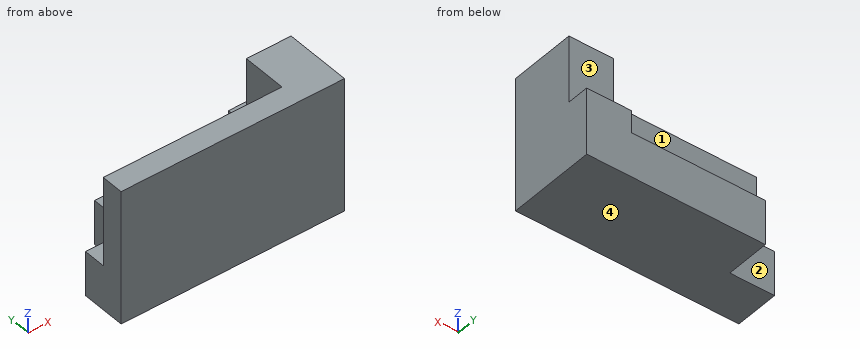
from build123d import *

# Parameters (mm, degrees)
SALIENTE_EXTRUIR1_DEPTH = 10
CROQUIS1_3_W            = 20
CROQUIS1_3_H            = 30
SALIENTE_EXTRUIR2_DEPTH = 30
SALIENTE_EXTRUIR3_DEPTH = 40
CROQUIS1_5_W            = 20
CROQUIS1_5_H            = 20
SALIENTE_EXTRUIR4_DEPTH = 20


with BuildPart() as part:
    # Croquis1 → Saliente-Extruir1 (new body)
    with BuildSketch(Plane(origin=(0, 0, 0), x_dir=(1, 0, 0), z_dir=(0, 1, 0))):
        Polygon((-30, 10), (-50, 10), (-50, -30), (30, -30), (30, 0), (30, 10), align=None)
    extrude(amount=SALIENTE_EXTRUIR1_DEPTH)

    # Croquis1<3> → Saliente-Extruir2 (add)
    with BuildSketch(Plane(origin=(0, 0, 0), x_dir=(1, 0, 0), z_dir=(0, 1, 0))):
        with Locations((40, -15)):
            Rectangle(CROQUIS1_3_W, CROQUIS1_3_H)
    extrude(amount=SALIENTE_EXTRUIR2_DEPTH)

    # Croquis1<4> → Saliente-Extruir3 (add)
    with BuildSketch(Plane(origin=(0, 0, 0), x_dir=(1, 0, 0), z_dir=(0, 1, 0))):
        Polygon((30, 30), (-30, 30), (-30, 10), (30, 10), (30, 0), (50, 0), (50, 30), align=None)
    extrude(amount=SALIENTE_EXTRUIR3_DEPTH)

    # Croquis1<5> → Saliente-Extruir4 (add)
    with BuildSketch(Plane(origin=(0, 0, 0), x_dir=(1, 0, 0), z_dir=(0, 1, 0))):
        with Locations((-40, 20)):
            Rectangle(CROQUIS1_5_W, CROQUIS1_5_H)
    extrude(amount=SALIENTE_EXTRUIR4_DEPTH)


solid = part.part
Part model, mm, in its own coordinate system. Face numbers are marked on the shaded views. A direction names the side the tool comes from. Coordinates: 2 decimals unless noted, no trailing zeros. Order: outer loops, then holes, each group sorted by start corner. A loop starts at its lowest first (then second) coordinate and runs counter-clockwise, first axis right, second up. Notation, with made-up numbers: (11, -7) - (21, -7) arc R22 ccw to (21, 24) - close; hole circle Ø5 at (-2.5, 16). An arc over 180 degrees is marked (long way). Use CSV: the item, a comma, the result in double quotes.
Item 1: Drop flat-ended pins along their axis: P1, Ø12, axis at x = -27.5, z = 15, coming from the +Y side; P2, Ø10, axis at x = 17, y = 26, coming from the +Z side; P3, Ø22, axis at x = 41.5, z = 12, coming from the +Y side. Give the stop position or say it passes through.
Solved:
P1,"stops at y = 10"
P2,"stops at z = -10"
P3,"stops at y = 30"
Item 2: Saw through at A-A on x = -42.5. Give the cut face in (y, z).
Solved:
outline,"(0, -30) - (20, -30) - (20, -10) - (10, -10) - (10, 30) - (0, 30) - close"
Item 3: Probe probe 1 along X at (y, z) = (28, -2.5); probe 2 along Y at (x, z) = (10, -5); probe 3 along Z at (x, y) = (25.5, 38). List the from-to ranges inside material, lowest first.
Solved:
probe 1,"x = 30 to 50"
probe 2,"y = 0 to 10"
probe 3,"z = -30 to -10"
Item 4: Saw through at B-B on y = 36. Give the cut face in (x, z), and give its area (3 significant figures).
Solved:
outline,"(-30, -30) - (50, -30) - (50, 0) - (30, 0) - (30, -10) - (-30, -10) - close"
area,"1,800 mm²"
Item 5: 3-axis set-ups, long thin cutter, end or side, ignore diameter. For the marked faces 1, 2, 3 and 4: which of +Z, -Z, +X, -X, +Y, -Y reach the whole face in a straight line?
Solved:
face 1,"+Z, -X, +Y"
face 2,"+Z, -Z, -X, +Y"
face 3,"+Z, +X, -X, +Y"
face 4,"-Z, +X, -X, +Y, -Y"
